Design review of the part built by this model. Coordinates are the model's own, in mm. Round coordinates to 2 decimals unless told otherwise and drop trailing zeros. Write each loop counter-clockwise with the first axis right and the second up, starting at its lowest first coordinate (ties: lowest second). Pieces come first, ordered by that corner, then holes. Notation, with made-up numbers: M 18,-31 L 54,-31 A16 cw 54,-21 Z; hole C 1.5,47.5 d8. An arc over 180 degrees is marked long. Use CSV: the item, a comma, the result in double quotes.
from build123d import *

# Parameters (mm, degrees)
BOSS_EXTRUDE1_DEPTH = 9
SKETCH2_R           = 4.5
CUT_EXTRUDE1_DEPTH  = 9


with BuildPart() as part:
    # Sketch1 → Boss-Extrude1 (new body)
    with BuildSketch(Plane(origin=(0, 0, 0), x_dir=(1, 0, 0), z_dir=(0, 1, 0))):
        Polygon((0, 9), (-7.794228634, 4.5), (-7.794228634, -4.5), (0, -9), (7.794228634, -4.5), (7.794228634, 4.5), align=None)
    extrude(amount=BOSS_EXTRUDE1_DEPTH)

    # Sketch2 → Cut-Extrude1 (cut)
    with BuildSketch(Plane(origin=(0, 9, 0), x_dir=(1, 0, 0), z_dir=(0, 1, 0))):
        with Locations(Location((0, 0, 0), (0, 0, 270))):  # turned: the seam where the file's is
            Circle(SKETCH2_R)
    extrude(amount=-CUT_EXTRUDE1_DEPTH, mode=Mode.SUBTRACT)


solid = part.part
1) Add section B-B on y = 5. Write out the cut boundary in (x, z).
Answers:
outline,"M -7.79,-4.5 L 0,-9 L 7.79,-4.5 L 7.79,4.5 L 0,9 L -7.79,4.5 Z; hole C 0,0 d9"
2) Wall thickness on line 1 along X through (y, z) = (3.25, 0); line 2 along Z through (x, y) = (3.5, 6); line 3 along Z through (x, y) = (-4, 3.25): over which ranges is each line inside the solid? List them lowest first. Write a range as [from, to].
Answers:
line 1,"[-7.79, -4.5], [4.5, 7.79]"
line 2,"[-6.98, -2.83], [2.83, 6.98]"
line 3,"[-6.69, -2.06], [2.06, 6.69]"
3) Add section C-C on x = 3.25. Write out the cut boundary in (y, z), then the cut area to 3 significant figures.
Answers:
outline,"M 0,-7.12 L 9,-7.12 L 9,-3.11 L 0,-3.11 Z; M 0,3.11 L 9,3.11 L 9,7.12 L 0,7.12 Z"
area,"72.2 mm²"
4) Add section A-A on z = 0. Write out the cut boundary in (x, y), then the cut area to 3 significant figures.
Answers:
outline,"M -7.79,0 L -4.5,0 L -4.5,9 L -7.79,9 Z; M 4.5,0 L 7.79,0 L 7.79,9 L 4.5,9 Z"
area,"59.3 mm²"
5) For pin 1 Ø1 at (x, y) = (3, 1) entering from +Z; pin 2 Ø1.5 at (x, y) = (6, 1.5) entering from -Z; pin 3 Ø3 at (x, y) = (5.5, 1) entering from -Z, all flat-tipped, find the tip position at first contact; note any pin that passes through.
Answers:
pin 1,"z = 7.56"
pin 2,"z = -5.97"
pin 3,"z = -6.69"
6) The part is to be moulded in two halves that separate along Z. For faces 1 (the face through (3.95, 4.44, -6.72)), 2 (the face through (-3.95, 4.44, 6.72)), 3 (the face through (7.794, 4, 0)), 4 (the face through (1.352, 4.563, 4.292)), say which applies: released by +Z, released by -Z, zero draft, split by the parting line, or undercut.
Answers:
face 1,"released by -Z"
face 2,"released by +Z"
face 3,"zero draft"
face 4,"undercut"
7) Add section D-D on z = 5.75. Write out the cut boundary in (x, y).
Answers:
outline,"M -5.63,0 L 5.63,0 L 5.63,9 L -5.63,9 Z"
